Drawing for the job (mm, zero at the part's lowest x, y, z). A direction names the side the tool comes from. Coordinates: 2 decimals unless noted, no trailing zeros. Order: outer loops, then holes, each group sorted by start corner. A loop starts at its lowest first (then second) coordinate and runs counter-clockwise, first axis right, second up.
1) Cut at C-C (z = 8). List the corners of the cut face in (x, y), and give its area (3 significant figures).
2) Pin check, flat tips, straight feed: pin 1 Ø1.5 at (y, z) = (17, 15) entering from +X; pin 2 Ø5 at (y, z) = (17, 31.5) entering from +X; pin 3 Ø8 at (x, z) = (11, 64.5) entering from +Y. Stop position of each tip, or through.
3) Tool access for the marked faces 1 and 2: list every direction of +Z, -Z, +X, -X, +Y, -Y with a clear straight run to the whole face (end or side of a thin tool).
4) Wall check: L1, parallel to Z at x = 31, y = 26.5; L2, parallel to Y at x = 12, z = 37; L3, parallel to X at y = 17.5, z = 5.5. Give the ranges that are in metal, low to high.
5) Cut at D-D (x = 4). List the corners of the cut face in (y, z).
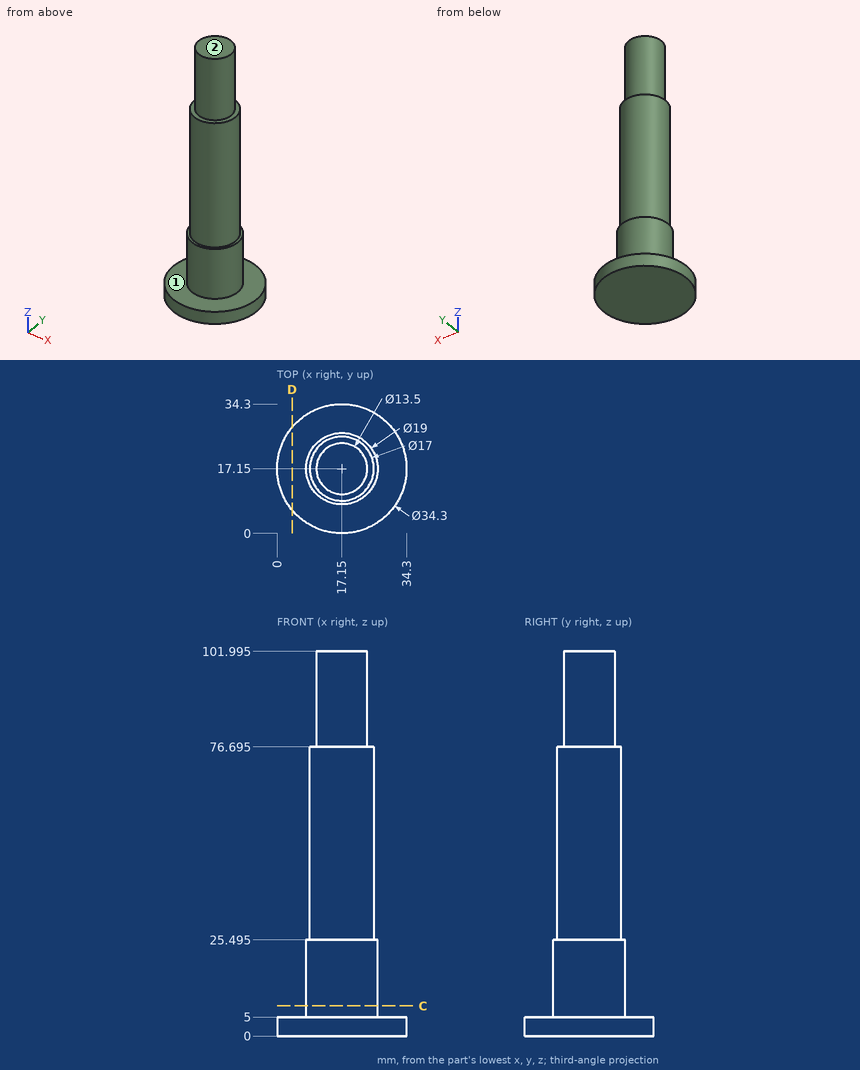
Geometry check:
1. outline: circle Ø19 at (17.15, 17.15)
1. area: 284 mm2
2. pin 1: stops at x = 26.65
2. pin 2: stops at x = 25.65
2. pin 3: stops at y = 25.37
3. face 1: +Z
3. face 2: +Z, +X, -X, +Y, -Y
4. L1: z = 0 to 5
4. L2: y = 10.39 to 23.91
4. L3: x = 7.66 to 26.64
5. outline: (6.14, 0) - (28.16, 0) - (28.16, 5) - (6.14, 5) - close
